Geometry check sheet. Reference: the model listing, model coordinates, mm. Face numbers are marked on the shaded views. Round coordinates to 2 decimals unless told otherwise and drop trailing zeros. Write each loop counter-clockwise with the first axis right and the second up, starting at its lowest first coordinate (ties: lowest second). Pieces come first, ordered by that corner, then holes. Notation, with made-up numbers: M 83.5,55.25 L 135.5,55.25 A31 ccw 135.5,84.25 Z; hole C 28.5,-14.75 d3. An arc over 180 degrees is marked long. One line per item, written item: value. Start each with the question number.
1. Section check A-A (x = 0). Record the boundary of the cut face in (y, z).
2. Scan lines: probe 1 along Z at (x, y) = (-4, 3.25); probe 2 along X at (y, z) = (3.25, 55); probe 3 along Z at (x, y) = (3.5, -2). Record each from-to range of solid material in increasing order. Write a range as [from, to].
3. Section check C-C (y = 7). Record the boundary of the cut face in (x, z).
4. Depth check by flat-ended pin: P1, Ø8, axis at y = -2.5, z = 44, coming from the +X side; P2, Ø1.9, axis at x = 3, y = 0, coming from the +Z side; P3, Ø6, axis at y = -6, z = 35, coming from the -X side. Enter the tip coordinate at first touch or a pass-through.
5. Release check for a two-part mould opening along X. For the marked faces 1 and 2 record: pulls with the +X half, pulls with the -X half, needs draft (parallel to the pull), parting line crosses it, or undercut.
6. Section check B-B (z = 27). Record the boundary of the cut face in (x, y).
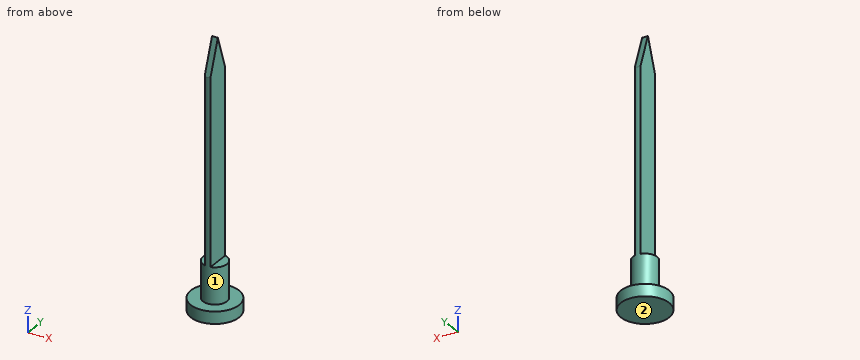
from build123d import *

# Parameters (mm, degrees)
F0_R     = 5
F1_DEPTH = 125
F2_W     = 7.022222
F2_H     = 110
F3_DEPTH = 12.5
F6_DEPTH = 12.5
F0_R_2   = 10
F8_DEPTH = 5


with BuildPart() as f1:
    # F0 (on Top) → F1 (new body)
    with BuildSketch(Plane.XY):
        Circle(F0_R)
    extrude(amount=F1_DEPTH)


with BuildPart() as f3:
    # F2 (on Front) → F3 (new body, symmetric)
    with BuildSketch(Plane.XZ):
        with Locations((-4.711111, 75)):
            Rectangle(F2_W, F2_H)
        with Locations((4.711111, 75)):
            Rectangle(F2_W, F2_H)
    extrude(amount=F3_DEPTH, both=True)


with BuildPart() as f1_1:
    add(f1.part)

    # F4: cut F3
    add(f3.part, mode=Mode.SUBTRACT)


with BuildPart() as f6:
    # F5 (on Right) → F6 (new body, symmetric)
    with BuildSketch(Plane.YZ):
        Polygon((32.54493, 130), (-35.225107, 130), (-35.607988, 80), (-10.720685, 80), (0, 110), (10.337801, 80), (32.54493, 80), align=None)
    extrude(amount=F6_DEPTH, both=True)


with BuildPart() as f1_2:
    add(f1_1.part)

    # F7: cut F6
    add(f6.part, mode=Mode.SUBTRACT)

    # F0 (on Top) → F8 (join)
    with BuildSketch(Plane.XY):
        Circle(F0_R_2)
        Circle(F0_R, mode=Mode.SUBTRACT)
    extrude(amount=F8_DEPTH)


solid = f1_2.part
Result sheet:
1. outline: M -10,0 L 10,0 L 10,5 L 5,5 L 5,95.49 L 0,110 L -5,96.01 L -5,5 L -10,5 Z
2. probe 1: z = [0, 5]
2. probe 2: x = [-1.2, 1.2]
2. probe 3: z = [0, 20]
3. outline: M -7.14,0 L 7.14,0 L 7.14,5 L -7.14,5 Z
4. P1: stops at x = 1.2
4. P2: stops at z = 20
4. P3: stops at x = -1.2
5. face 1: parting line crosses it
5. face 2: needs draft
6. outline: M -1.2,-4.85 A5 ccw 1.2,-4.85 L 1.2,4.85 A5 ccw -1.2,4.85 Z
